Check sheet for the modelled part. Datum: model origin and axes. Units: mm. A direction names the side the tool comes from. Round coordinates to 2 decimals unless told otherwise and drop trailing zeros. Loops run counter-clockwise (first coordinate to the right, second up) from the corner with the lowest first, then second, coordinate; pieces in that order, holes last. Notation, with made-up numbers: (81, 77.25) - (91, 77.25) arc R22 cw to (91, 102.25) - close; hole circle Ø4 at (87, -25). An arc over 180 degrees is marked (long way). Put each result on its own line as item: value.
```python
from build123d import *

# Parameters (mm, degrees)
SKETCH2_R                                        = 16
BOSS_EXTRUDE1_DEPTH                              = 8
SKETCH3_W                                        = 27.624731793
SKETCH3_H                                        = 2
SKETCH3_W_2                                      = 37.15735793
SKETCH3_W_3                                      = 33.69266167
SKETCH3_W_4                                      = 12.751314483
CUT_EXTRUDE1_DEPTH                               = 6
SKETCH4_R                                        = 2.5
CUT_EXTRUDE2_DEPTH                               = 4
TAP_DRILL_FOR_M3X0_5_TAP1_D                      = 2.5
TAP_DRILL_FOR_M3X0_5_TAP1_DEPTH                  = 5.5
TAP_DRILL_FOR_M3X0_5_TAP1_TIP                    = 0.751075774
SKETCH8_R                                        = 9
SKETCH8_R_2                                      = 8
BOSS_EXTRUDE2_DEPTH                              = 0.5
CBORE_FOR_M4_PAN_HEAD_MACHINE_SCREW1_D           = 2.5
CBORE_FOR_M4_PAN_HEAD_MACHINE_SCREW1_DEPTH       = 8.001
CBORE_FOR_M4_PAN_HEAD_MACHINE_SCREW1_CBORE_D     = 4
CBORE_FOR_M4_PAN_HEAD_MACHINE_SCREW1_CBORE_DEPTH = 4
CIRPATTERN1_COUNT                                = 4
CUT_EXTRUDE3_DEPTH                               = 20.25


with BuildPart() as part:
    # Sketch2 → Boss-Extrude1 (new body)
    with BuildSketch(Plane(origin=(0, 0, 0), x_dir=(1, 0, 0), z_dir=(0, 1, 0))):
        with Locations(Location((0, 0, 0), (0, 0, 270))):  # turned: the seam where the file's is
            Circle(SKETCH2_R)
    extrude(amount=BOSS_EXTRUDE1_DEPTH)

    # Sketch3 → Cut-Extrude1 (cut)
    with BuildSketch(Plane(origin=(0, 8, 0), x_dir=(1, 0, 0), z_dir=(0, 1, 0))):
        with Locations((0.605596929, -12)):
            Rectangle(SKETCH3_W, SKETCH3_H)
        with Locations((-0.172635518, 4)):
            Rectangle(SKETCH3_W_2, SKETCH3_H)
        with Locations((-0.604755395, 8)):
            Rectangle(SKETCH3_W_3, SKETCH3_H)
        with Locations((0.605596929, 12)):
            Rectangle(SKETCH3_W, SKETCH3_H)
        with Locations((-0.604755395, -8)):
            Rectangle(SKETCH3_W_3, SKETCH3_H)
        with Locations((-0.172635518, -4)):
            Rectangle(SKETCH3_W_2, SKETCH3_H)
        with Locations((-12.375657242, 0)):
            Rectangle(SKETCH3_W_4, SKETCH3_H)
        with Locations((12.375657242, 0)):
            Rectangle(SKETCH3_W_4, SKETCH3_H)
    extrude(amount=-CUT_EXTRUDE1_DEPTH, mode=Mode.SUBTRACT)

    # Sketch4 → Cut-Extrude2 (cut)
    with BuildSketch(Plane(origin=(0, 8, 0), x_dir=(1, 0, 0), z_dir=(0, 1, 0))):
        with Locations(Location((0, 0, 0), (0, 0, 270))):  # turned: the seam where the file's is
            Circle(SKETCH4_R)
    extrude(amount=-CUT_EXTRUDE2_DEPTH, mode=Mode.SUBTRACT)

    # Tap Drill for M3x0.5 Tap1
    with Locations(Plane(origin=(0, 0, 0), x_dir=(-1, 0, 0), z_dir=(0, -1, 0))):
        with Locations((0, 0)):
            Hole(TAP_DRILL_FOR_M3X0_5_TAP1_D / 2, depth=TAP_DRILL_FOR_M3X0_5_TAP1_DEPTH)
            with Locations((0, 0, -(TAP_DRILL_FOR_M3X0_5_TAP1_DEPTH + TAP_DRILL_FOR_M3X0_5_TAP1_TIP / 2))):  # 118° drill point
                Cone(0, TAP_DRILL_FOR_M3X0_5_TAP1_D / 2, TAP_DRILL_FOR_M3X0_5_TAP1_TIP, mode=Mode.SUBTRACT)

    # Sketch8 → Boss-Extrude2 (add)
    with BuildSketch(Plane.XZ):
        with Locations(Location((0, 0, 0), (0, 0, 90))):  # turned: the seam where the file's is
            Circle(SKETCH8_R)
        with Locations(Location((0, 0, 0), (0, 0, 270))):  # turned: the seam where the file's is
            Circle(SKETCH8_R_2, mode=Mode.SUBTRACT)
    extrude(amount=BOSS_EXTRUDE2_DEPTH)

    # CBORE for M4 Pan Head Machine Screw1
    with Locations(Plane(origin=(0, 8, 0), x_dir=(1, 0, 0), z_dir=(0, 1, 0))):
        with Locations((-8.1, -8.1)):
            cbore_for_m4_pan_head_machine_screw1 = CounterBoreHole(CBORE_FOR_M4_PAN_HEAD_MACHINE_SCREW1_D / 2, CBORE_FOR_M4_PAN_HEAD_MACHINE_SCREW1_CBORE_D / 2, CBORE_FOR_M4_PAN_HEAD_MACHINE_SCREW1_CBORE_DEPTH, depth=CBORE_FOR_M4_PAN_HEAD_MACHINE_SCREW1_DEPTH)

    # CirPattern1: CBORE for M4 Pan Head Machine Screw1 ×4 about axis
    cirpattern1_axis = Axis((0, 0, 0), (0, 1, 0))
    for i in range(1, CIRPATTERN1_COUNT):
        add(cbore_for_m4_pan_head_machine_screw1.rotate(cirpattern1_axis, i * 360 / CIRPATTERN1_COUNT), mode=Mode.SUBTRACT)

    # Sketch12 → Cut-Extrude3 (cut, symmetric)
    with BuildSketch(Plane(origin=(0, 0, 0), x_dir=(0, 0, -1), z_dir=(1, 0, 0))):
        Polygon((0, 8), (16, 8), (17.032384138, 8), (17.032384138, 4.379654991), align=None)
    cut_extrude3 = extrude(amount=CUT_EXTRUDE3_DEPTH, both=True, mode=Mode.SUBTRACT)

    # Mirror1: Cut-Extrude3 across plane
    add(cut_extrude3.mirror(Plane.XY), mode=Mode.SUBTRACT)


solid = part.part
```
Item 1: Section check C-C on x = 12.5. Enter the section's corners in (y, z), then the cut area to 3 significant figures.
Filled sheet:
outline: (0, -9.99) - (5.88, -9.99) - (6.09, -9) - (2, -9) - (2, -7) - (6.51, -7) - (6.94, -5) - (2, -5) - (2, -3) - (7.36, -3) - (7.79, -1) - (2, -1) - (2, 1) - (7.79, 1) - (7.36, 3) - (2, 3) - (2, 5) - (6.94, 5) - (6.51, 7) - (2, 7) - (2, 9) - (6.09, 9) - (5.88, 9.99) - (0, 9.99) - close
area: 89.0 mm²
Item 2: Go/stop test with flat-tipped pins: pin 1 (2 mm diameter, centred on x = 8, y = 5, fed in from -Z); pin 2 (2 mm diameter, centred on x = -3, z = -4.5, fed in from +Y); pin 3 (6 mm diameter, centred on x = 0, z = 0, fed in from -Y); pin 4 (5.5 mm diameter, centred on x = -1, z = 1, fed in from +Y). Record where each tip stops, or that it passes through.
Filled sheet:
pin 1: z = -14.39
pin 2: y = 6.94
pin 3: y = 0
pin 4: y = 8
Item 3: Section check B-B on x = -10.5. Enter the section's corners in (y, z).
Filled sheet:
outline: (0, -12.07) - (2, -12.07) - (2, -11) - (5.66, -11) - (6.09, -9) - (2, -9) - (2, -7) - (6.51, -7) - (6.94, -5) - (2, -5) - (2, -3) - (7.36, -3) - (7.79, -1) - (2, -1) - (2, 1) - (7.79, 1) - (7.36, 3) - (2, 3) - (2, 5) - (6.94, 5) - (6.51, 7) - (2, 7) - (2, 9) - (6.09, 9) - (5.66, 11) - (2, 11) - (2, 12.07) - (0, 12.07) - close
Item 4: Tool access check on faces 4 (the flat face through (11, 4, 9)), 5 (the flat face through (6, 5, 0)), 6 (the cylindrical face through (7.72, 1.53, 9.29)), 7 (the flat face through (-8.1, 4, 9.5)). Record the directions out of +Z, -Z, +X, -X, +Y, -Y that give a thin tool (end or side, any length) a straight path to the whole face; none if there is none.
Filled sheet:
face 4: +X, -X, +Y
face 5: +X, +Y
face 6: +Y, -Y
face 7: +Y
Item 5: Release check for a two-part mould opening along Z. For faces 1 (the flat face through (3.772, 7.606, 1.854)), 2 (the flat face through (3.772, 7.606, -1.854)), 3 (the flat face through (-6, 5, 0)) record: +Z half, -Z half, draft (parallel to the pull), parting line (faces both ways), or undercut.
Filled sheet:
face 1: +Z half
face 2: -Z half
face 3: undercut
Item 6: Thickness scan on line 1 (Z direction, x = 14, y = 5.75); line 2 (Z direction, x = 0, y = 1); line 3 (Z direction, x = 8.1, y = 1.1). Record the ranges inside material, lowest first. Write a range as from..to.
Filled sheet:
line 1: -7..-5, -3..-1, 1..3, 5..7
line 2: -16..-1.25, 1.25..16
line 3: -13.8..-9.35, -6.85..6.85, 9.35..13.8
Item 7: Section check A-A on y = 0.5. Enter the section's corners in (x, z).
Filled sheet:
outline: circle Ø32 at (0, 0); hole circle Ø2.5 at (-8.1, -8.1); hole circle Ø2.5 at (-8.1, 8.1); hole circle Ø2.5 at (0, 0); hole circle Ø2.5 at (8.1, -8.1); hole circle Ø2.5 at (8.1, 8.1)
